Design review of the part shown in the three views and the two pictorial views. Dimensions are in mm from the part's minimum x, y and z. Give positions to 0.01 mm unless a question says otherwise; leave off trailing zeros. Write each loop counter-clockwise with the first axis right and the second up, starting at its lowest first coordinate (ties: lowest second). Pieces come first, ordered by that corner, then holes. Notation, with made-up numbers: M 13.5,62.25 L 32.5,62.25 A12 ccw 32.5,76.25 Z; hole C -16.75,-9 d4. An arc over 180 degrees is marked long. Write item = value, one per line.
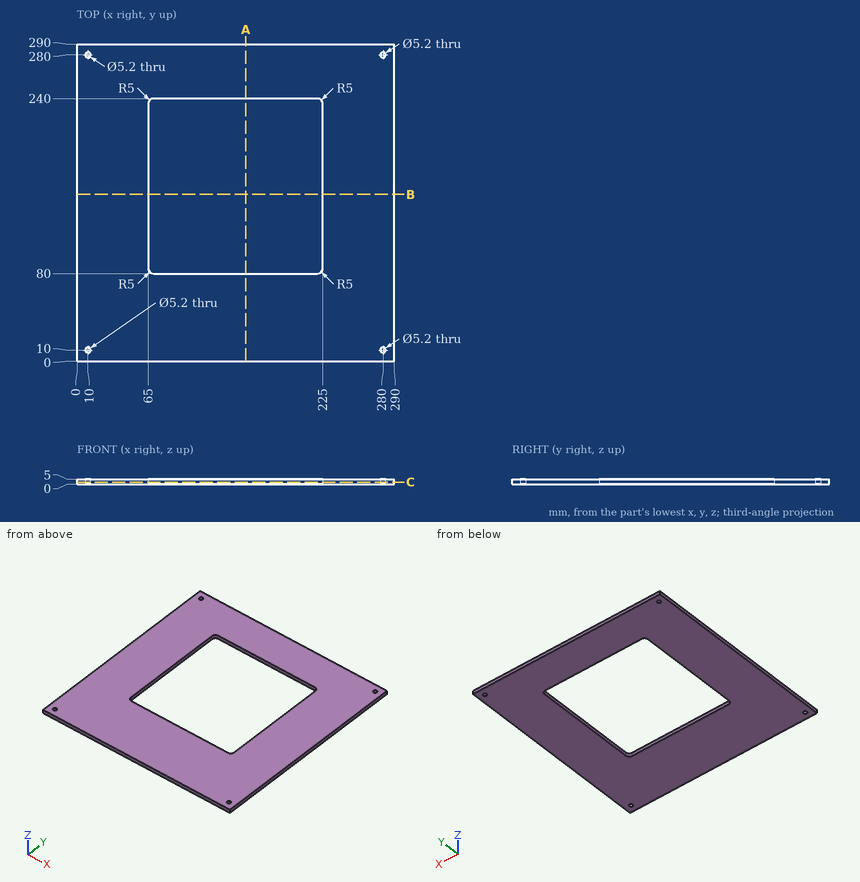
1. For line 1 along X through (y, z) = (280, 2.2); line 2 along Y through (x, z) = (174.5, 3.35), list the stretches that pass through material, from the lowest coordinate up. Write a range as from..to.
Responses:
line_1 = 0..7.4, 12.6..277.4, 282.6..290
line_2 = 0..80, 240..290
2. We need section B-B, the plane y = 152.5. Write out the cut boundary in (x, z).
Responses:
outline = M 0,0 L 65,0 L 65,5 L 0,5 Z; M 225,0 L 290,0 L 290,5 L 225,5 Z
3. We need section C-C, the plane z = 2.1. Write out the cut boundary in (x, y), then the cut area to 3 significant figures.
Responses:
outline = M 0,0 L 290,0 L 290,290 L 0,290 Z; hole C 10,10 d5.2; hole C 10,280 d5.2; hole M 65,85 A5 ccw 70,80 L 220,80 A5 ccw 225,85 L 225,235 A5 ccw 220,240 L 70,240 A5 ccw 65,235 Z; hole C 280,10 d5.2; hole C 280,280 d5.2
area = 58,400 mm2
4. We need section A-A, the plane x = 154.5. Write out the cut boundary in (y, z), then the cut area to 3 significant figures.
Responses:
outline = M 0,0 L 80,0 L 80,5 L 0,5 Z; M 240,0 L 290,0 L 290,5 L 240,5 Z
area = 650 mm2
